```python
from build123d import *

# Parameters (mm, degrees)
BOSS_EXTRU_1_DEPTH                                 = 40
CHAMBRAGE_POUR_VIS_T_TE_HEXAGONALE_M51_D           = 5.5
CHAMBRAGE_POUR_VIS_T_TE_HEXAGONALE_M51_CBORE_D     = 10
CHAMBRAGE_POUR_VIS_T_TE_HEXAGONALE_M51_CBORE_DEPTH = 5.4


with BuildPart() as part:
    # Esquisse1 → Boss.-Extru.1 (new body)
    with BuildSketch(Plane.XY):
        Polygon((-10, 0.691167323), (8.452994616, 0.691167323), (20, 20.691167323), (-10, 20.691167323), align=None)
    extrude(amount=BOSS_EXTRU_1_DEPTH)

    # Chambrage pour vis à tête hexagonale M51 (through all)
    with Locations(Plane(origin=(0, 20.691167323, 0), x_dir=(1, 0, 0), z_dir=(0, 1, 0))):
        with Locations((0, -20)):
            CounterBoreHole(CHAMBRAGE_POUR_VIS_T_TE_HEXAGONALE_M51_D / 2, CHAMBRAGE_POUR_VIS_T_TE_HEXAGONALE_M51_CBORE_D / 2, CHAMBRAGE_POUR_VIS_T_TE_HEXAGONALE_M51_CBORE_DEPTH)


solid = part.part
```
Geometry: final body of the model. Coordinates: model frame, mm. A direction names the side the tool comes from. Coordinates: 2 decimals unless noted, no trailing zeros. Loops run counter-clockwise (first coordinate to the right, second up) from the corner with the lowest first, then second, coordinate; pieces in that order, holes last. Notation, with made-up numbers: M 18.5,62 L 48.5,62 A15 cw 48.5,87 Z; hole C 31,-26.5 d11. An arc over 180 degrees is marked long. Put each result on its own line as item: value.
(1) Material intervals for probe 1 along Z at (x, y) = (0, 19.15); probe 2 along X at (y, z) = (19.5, 20); probe 3 along Z at (x, y) = (0, 4.75), sorted ascending.
Answer sheet:
probe 1: z = 0 to 15, 25 to 40
probe 2: x = -10 to -5, 5 to 19.31
probe 3: z = 0 to 17.25, 22.75 to 40
(2) Cut plane D-D on z = 24. Return the cut outline in (x, y), then the cut area to 3 significant figures.
Answer sheet:
outline: M -10,0.69 L 8.45,0.69 L 20,20.69 L 3,20.69 L 3,15.29 L -3,15.29 L -3,20.69 L -10,20.69 Z
area: 452 mm^2
(3) Cut plane B-B on x = 0. Return the cut outline in (y, z), then the cut area to 3 significant figures.
Answer sheet:
outline: M 0.69,0 L 20.69,0 L 20.69,15 L 15.29,15 L 15.29,17.25 L 0.69,17.25 Z; M 0.69,22.75 L 15.29,22.75 L 15.29,25 L 20.69,25 L 20.69,40 L 0.69,40 Z
area: 666 mm^2
(4) Access query for faces 5 (the face through (-1.08, 18.03, 24.88)), 6 (the face through (1, 11, 0)). Directions: +Z, -Z, +X, -X, +Y, -Y. A direction counts if a zero-diameter tool reaches every point of the face in a straight line with its end or side. Return the directions, or none.
Answer sheet:
face 5: +Y
face 6: -Z, +X, -X, +Y, -Y
(5) Cut plane C-C on x = -4. Return the cut outline in (y, z), then the cut area to 3 significant figures.
Answer sheet:
outline: M 0.69,0 L 20.69,0 L 20.69,17 L 15.29,17 L 15.29,23 L 20.69,23 L 20.69,40 L 0.69,40 Z
area: 768 mm^2
(6) Draft query along Z for faces 1 (the face through (2.2, 15.291, 22.2)), 2 (the face through (0.358, 7.889, 17.273)), 3 (the face through (-10, 11, 20)), 4 (the face through (1, 11, 40)). Return one class per face: pulls with the +Z half, pulls with the -Z half, needs draft (parallel to the pull), parting line crosses it, or undercut.
Answer sheet:
face 1: undercut
face 2: undercut
face 3: needs draft
face 4: pulls with the +Z half
(7) Cut plane A-A on z = 20. Return the cut outline in (x, y), then the cut area to 3 significant figures.
Answer sheet:
outline: M -10,0.69 L -2.75,0.69 L -2.75,15.29 L -5,15.29 L -5,20.69 L -10,20.69 Z; M 2.75,0.69 L 8.45,0.69 L 20,20.69 L 5,20.69 L 5,15.29 L 2.75,15.29 Z
area: 350 mm^2
(8) First-contact query: pin 1 (4.5 mm diameter, centred on x = 0, z = 20, fed in from +Y); pin 2 (5 mm diameter, centred on y = 6.5, z = 34, fed in from +X); pin 3 (8 mm diameter, centred on y = 7.5, z = 32, fed in from +X); pin 4 (6 mm diameter, centred on y = 2.5, z = 30, fed in from +X). Flat tips, straight axial feed; report the tip coordinate or a pass-through.
Answer sheet:
pin 1: passes through
pin 2: stops at x = 13.25
pin 3: stops at x = 14.69
pin 4: stops at x = 11.23
